from build123d import *

# Parameters (mm, degrees)
SKETCH_1_R      = 8
SKETCH_1_R_2    = 12
SKETCH_1_W      = 115
SKETCH_1_H      = 12
EXTRUDE_1_DEPTH = 12


with BuildPart() as part:
    # 草图1 → 凸台-拉伸1 (new body)
    with BuildSketch(Plane.XY):
        with Locations((115, 0)):
            Circle(SKETCH_1_R)
        Circle(SKETCH_1_R)
        with Locations((57.5, 0)):
            Circle(SKETCH_1_R_2)
        with Locations((57.5, 0)):
            Rectangle(SKETCH_1_W, SKETCH_1_H)
    extrude(amount=EXTRUDE_1_DEPTH)

    # 草图2 → 旋转2 (revolve)
    with BuildSketch(Plane(origin=(0, 0, 0), x_dir=(1, 0, 0), z_dir=(0, 1, 0))):
        with BuildLine():
            ThreePointArc((-8, 6.94427191), (-4.281865077, 9.210068308), (0, 10))
            Line((0, 10), (0, 0))
            Line((0, 0), (-8, 0))
            Line((-8, 0), (-8, 6.94427191))
        make_face()
    revolve_2 = revolve(axis=Axis((0, 0, -10), (0, 0, 1)))

    # 镜向1: 旋转2 across plane
    add(revolve_2.mirror(Plane(origin=(57.5, 0, 0), x_dir=(0, 0, 1), z_dir=(1, 0, 0))))

    # 草图3 → 旋转3 (revolve)
    with BuildSketch(Plane(origin=(0, 0, 0), x_dir=(1, 0, 0), z_dir=(0, 1, 0))):
        with BuildLine():
            Line((57.5, -12), (57.5, -13))
            ThreePointArc((57.5, -13), (52.022774425, -14.322921748), (47.753205655, -18))
            Line((47.753205655, -18), (45.5, -18))
            Line((45.5, -18), (45.5, -12))
            Line((45.5, -12), (57.5, -12))
        make_face()
    revolve(axis=Axis((57.5, 0, 12), (0, 0, 1)))


solid = part.part
Geometry check sheet. Reference: the model listing, model coordinates, mm. A direction names the side the tool comes from. Round coordinates to 2 decimals unless told otherwise and drop trailing zeros. Order: outer loops, then holes, each group sorted by start corner. A loop starts at its lowest first (then second) coordinate and runs counter-clockwise, first axis right, second up. Notation, with made-up numbers: (26.5, 4) -> (39.5, 4) arc R24 ccw to (39.5, 32) -> close; hole circle Ø8 at (50, 18). An arc over 180 degrees is marked (long way). Use one line per item in the form item = value.
1. Cross-section at D-D, the plane x = 115. Enter the section's corners in (y, z), plus the area to 3 significant figures.
Working result:
outline = (-8, -6.94) arc R12 ccw to (8, -6.94) -> (8, 12) -> (-8, 12) -> close
area = 337 mm^2
2. Go/stop test with flat-tipped pins: pin 1 (12 mm diameter, centred on x = 79.5, y = 2, fed in from -Z); pin 2 (5 mm diameter, centred on y = 3.5, z = -2.5, fed in from -X); pin 3 (6 mm diameter, centred on x = 89, z = -1, fed in from +Y). Record where each tip stops, or that it passes through.
Working result:
pin_1 = 0
pin_2 = -7.94
pin_3 = 6
3. Cross-section at B-B, the plane x = 57.5. Enter the section's corners in (y, z).
Working result:
outline = (-12, 0) -> (12, 0) -> (12, 18) -> (9.75, 18) arc R12 cw to (-9.75, 18) -> (-12, 18) -> close
4. Set-up check for faces 4 (the face through (26, 6, 6)), 5 (the face through (26, -6, 6)), 6 (the face through (57, -10, 18)): record each of +Z, -Z, +X, -X, +Y, -Y from which the full face is reachable in a straight line by a thin tool's end or side.
Working result:
face_4 = +Z, -Z, +Y
face_5 = +Z, -Z, -Y
face_6 = +Z, +X, -X, +Y, -Y
5. Cross-section at C-C, the plane y = 0. Enter the section's corners in (x, z), plus the area to 3 significant figures.
Working result:
outline = (-8, -6.94) arc R12 ccw to (8, -6.94) -> (8, 0) -> (107, 0) -> (107, -6.94) arc R12 ccw to (123, -6.94) -> (123, 12) -> (69.5, 12) -> (69.5, 18) -> (67.25, 18) arc R12 cw to (47.75, 18) -> (45.5, 18) -> (45.5, 12) -> (-8, 12) -> close
area = 1,940 mm^2
6. Scan lines: line 1 along X through (y, z) = (7.25, 1); line 2 along Z through (x, y) = (-2, -1.5); line 3 along Y through (x, z) = (38.5, 11). Record each from-to range of solid material in increasing order. Write a range as from..to.
Working result:
line_1 = -3.38..3.38, 47.94..67.06, 111.62..118.38
line_2 = -9.74..12
line_3 = -6..6
7. Cross-section at A-A, the plane z = 1.5. Enter the section's corners in (x, y).
Working result:
outline = (5.29, -6) -> (47.11, -6) arc R12 ccw to (67.89, -6) -> (109.71, -6) arc R8 ccw (long way) to (109.71, 6) -> (67.89, 6) arc R12 ccw to (47.11, 6) -> (5.29, 6) arc R8 ccw (long way) to start
8. Mould release check, pull along X, two halves, no side actions. Record for faces 1 (the face through (89, 6, 6)), 2 (the face through (95, 0, 12)), 3 (the face through (57, 0, 0)): pulls with the +X half, pulls with the -X half, needs draft (parallel to the pull), parting line crosses it, or undercut.
Working result:
face_1 = undercut
face_2 = needs draft
face_3 = undercut
